Source: CAD feature listing. Evaluate the final solid. Frame: model axes, mm. A direction names the side the tool comes from. Coordinates: 2 decimals unless noted, no trailing zeros. Write each loop counter-clockwise with the first axis right and the second up, starting at its lowest first coordinate (ties: lowest second). Pieces come first, ordered by that corner, then holes. Notation, with made-up numbers: M 36,27 L 59,27 A21 ccw 59,49 Z; hole C -14,50.5 d1. An arc over 180 degrees is marked long. Write item = value, one per line. Start each with the question number.
1. Pin query (flat end, axial travel): pin 1 Ø10 at (y, z) = (5.5, 5.5) entering from +X; pin 2 Ø3 at (x, z) = (-6, 5.5) entering from -Y; pin 3 Ø1.5 at (y, z) = (-3.5, 17.5) entering from +X. Return the tip coordinate at first contact, or that it passes through.
2. Section query C-C (z = 25.5). Output: boundary loops of the cut face in (x, y), then the cut area to 3 significant figures.
3. Access query for faces 1 (the face through (1.18, -2.26, 26.97)), 2 (the face through (0, 0, 0)). Directions: +Z, -Z, +X, -X, +Y, -Y. A direction counts if a zero-diameter tool reaches every point of the face in a straight line with its end or side. Return the directions, or none.
4. Line query: line 1 along Z through (x, y) = (-1.5, 2.25); line 2 along Z through (x, y) = (-4, 10); line 3 along Y through (x, z) = (0, 12). Output: solid intervals per line, ascending.
5. Section query A-A (y = 0). Output: boundary loops of the cut face in (x, z).
6. Section query D-D (z = 7.75). Output: boundary loops of the cut face in (x, y).
```python
from build123d import *

# Parameters (mm, degrees)
CROQUIS1_R              = 15
SALIENTE_EXTRUIR1_DEPTH = 25
REDONDEO2_R             = 5
CROQUIS2_R              = 2.55
SALIENTE_EXTRUIR2_DEPTH = 4


with BuildPart() as part:
    # Croquis1 → Saliente-Extruir1 (new body)
    with BuildSketch(Plane.XY):
        Circle(CROQUIS1_R)
    extrude(amount=SALIENTE_EXTRUIR1_DEPTH)

    # Redondeo2
    redondeo2_edges = [part.edges().sort_by_distance(p)[0] for p in [
        (-15, 0, 0),
        (-15, 0, 25),
    ]]
    fillet(redondeo2_edges, radius=REDONDEO2_R)

    # Croquis2 → Saliente-Extruir2 (add)
    with BuildSketch(Plane.XY.offset(25)):
        Circle(CROQUIS2_R)
    extrude(amount=SALIENTE_EXTRUIR2_DEPTH)


solid = part.part
```
Results are:
q1.pin_1 = 14.99
q1.pin_2 = -14.31
q1.pin_3 = 14.75
q2.outline = C 0,0 d5.1
q2.area = 20.4 mm^2
q3.face_1 = +Z
q3.face_2 = -Z, +X, -X, +Y, -Y
q4.line_1 = 0 to 25
q4.line_2 = 0.06 to 24.94
q4.line_3 = -15 to 15
q5.outline = M -15,5 A5 ccw -10,0 L 10,0 A5 ccw 15,5 L 15,20 A5 ccw 10,25 L 2.55,25 L 2.55,29 L -2.55,29 L -2.55,25 L -10,25 A5 ccw -15,20 Z
q6.outline = C 0,0 d30
